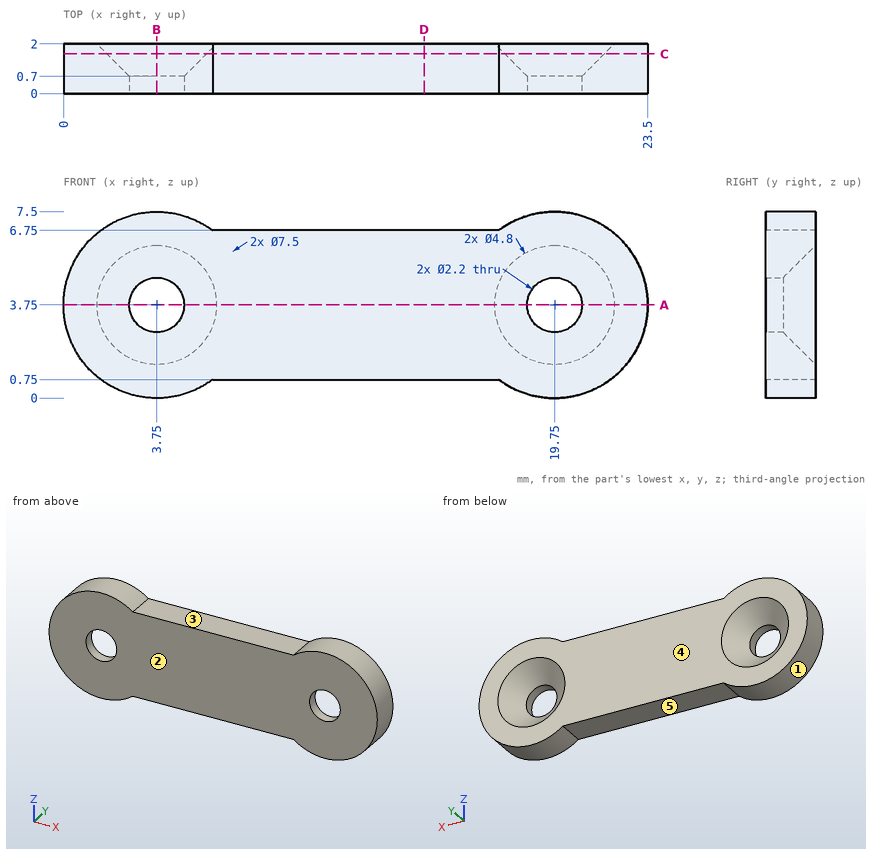
Answer from the drawing. Dimensions are ordinates in mm from the lowest x, y and z of the part. A direction names the side the tool comes from. Give positions to 0.01 mm unless a question says otherwise; leave off trailing zeros. Loops run counter-clockwise (first coordinate to the right, second up) from the corner with the lowest first, then second, coordinate; pieces in that order, holes last.
Item 1: A tool of negligible diameter and unlimited length cuts with its end or side. For the marked faces 3, 4 and 5, from which of +Z, -Z, +X, -X, +Y, -Y can it reach the whole face along a straight path? Write none if from no direction.
Derived:
face 3: +Z, +Y, -Y
face 4: +Z, -Z, +X, -X, +Y
face 5: -Z, +Y, -Y
Item 2: A cutting plane is placed at B-B (x = 3.75). Give the vertices of the cut face in (y, z), then the cut area to 3 significant figures.
Derived:
outline: (0, 0) - (2, 0) - (2, 1.35) - (0.7, 2.65) - (0, 2.65) - close; (0, 4.85) - (0.7, 4.85) - (2, 6.15) - (2, 7.5) - (0, 7.5) - close
area: 8.91 mm2
Item 3: A cutting plane is placed at C-C (y = 1.6). Give the vertices of the cut face in (x, z).
Derived:
outline: (6, 0.75) - (17.5, 0.75) arc R3.75 ccw (long way) to (17.5, 6.75) - (6, 6.75) arc R3.75 ccw (long way) to start; hole circle Ø4 at (3.75, 3.75); hole circle Ø4 at (19.75, 3.75)
Item 4: Find the intervals of material crossed by line 1 along X through (y, z) = (1.85, 2.25); line 2 along X through (y, z) = (1.25, 5); line 3 along Z through (x, y) = (12.75, 0.5), in increasing order.
Derived:
line 1: x = 0.31 to 2.07, 5.43 to 18.07, 21.43 to 23.19
line 2: x = 0.21 to 2.67, 4.83 to 18.67, 20.83 to 23.29
line 3: z = 0.75 to 6.75
Item 5: Determine the mould class of the marked faces 1 and 2 for opening direction X: +X half, -X half, draft (parallel to the pull), parting line (faces both ways), or undercut.
Derived:
face 1: undercut
face 2: draft
Item 6: Each of these flat-tipped pins is pushed along its axis until it touches: pin 1 Ø1.8 at (x, z) = (3.75, 3.75) entering from -Y (3 decimals); pin 2 Ø1 at (x, y) = (12.5, 1) entering from +Z. Where does it stop, or does it pass through?
Derived:
pin 1: passes through
pin 2: stops at z = 6.75
Item 7: A cutting plane is placed at A-A (z = 3.75). Give the vertices of the cut face in (x, y).
Derived:
outline: (0, 0) - (2.65, 0) - (2.65, 0.7) - (1.35, 2) - (0, 2) - close; (4.85, 0) - (18.65, 0) - (18.65, 0.7) - (17.35, 2) - (6.15, 2) - (4.85, 0.7) - close; (20.85, 0) - (23.5, 0) - (23.5, 2) - (22.15, 2) - (20.85, 0.7) - close
Item 8: A cutting plane is placed at D-D (x = 14.5). Give the vertices of the cut face in (y, z).
Derived:
outline: (0, 0.75) - (2, 0.75) - (2, 6.75) - (0, 6.75) - close
